For this review, use the dimensioned drawing (mm, ordinates from the lowest corner) and the shaded views. A direction names the side the tool comes from. Coordinates: 2 decimals unless noted, no trailing zeros. Loops run counter-clockwise (first coordinate to the right, second up) from the corner with the lowest first, then second, coordinate; pieces in that order, holes last. Notation, with made-up numbers: M 81,-29.5 L 126,-29.5 A8 ccw 126,-15.5 Z; hole C 9.25,64 d7. An arc over 180 degrees is marked long. Write item = value, one per line.
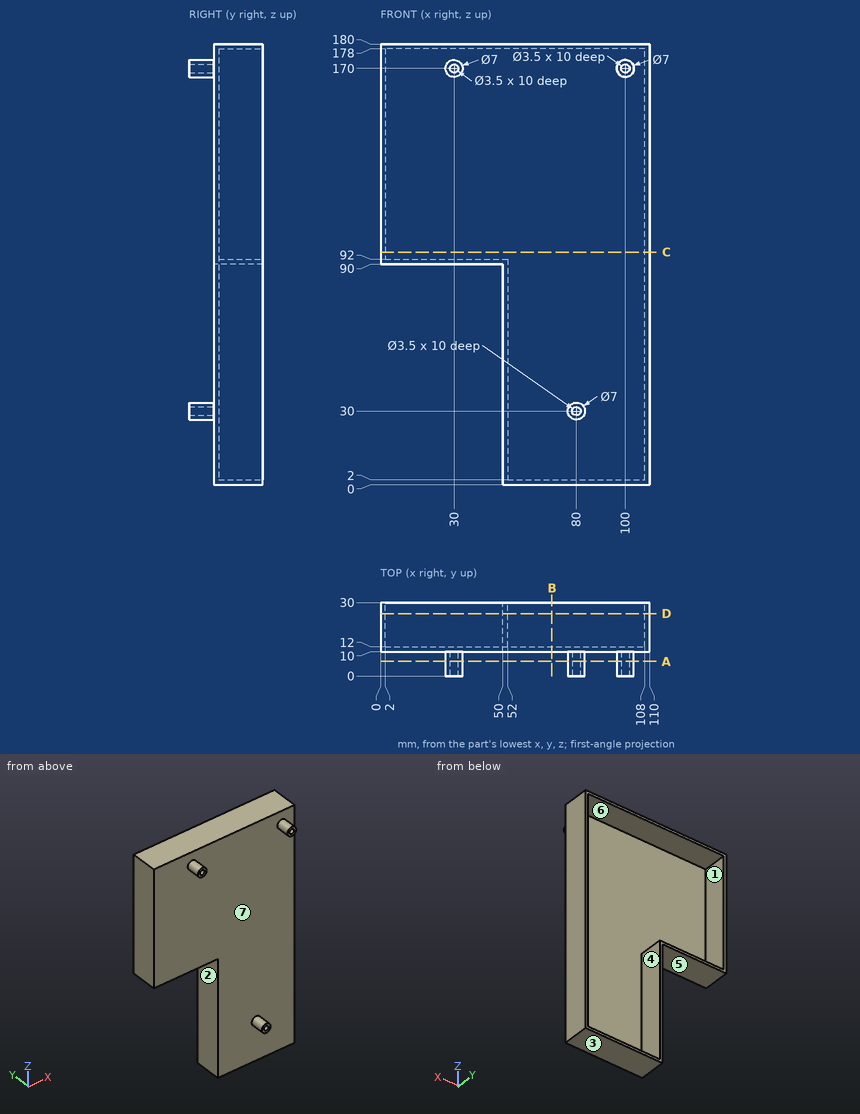
Q1. Machinability: for the marked faces 1, 2 and 3, which of the approach directions +Z, -Z, +X, -X, +Y, -Y give a long, thin tool a straight path to every point of the face, cutting with its end or side? Answer none if there is none.
Solved:
face_1 = +Y
face_2 = -Z, -X, +Y, -Y
face_3 = -Z, +X, -X, +Y, -Y
Q2. Add section D-D (y = 25.5). Write out the cut boundary in (x, z).
Solved:
outline = M 0,90 L 50,90 L 50,0 L 110,0 L 110,180 L 0,180 Z; hole M 2,92 L 52,92 L 52,2 L 108,2 L 108,178 L 2,178 Z
Q3. For pin 1 Ø1 at (x, z) = (80, 29.5) entering from -Y; pin 2 Ø4 at (x, z) = (30, 170) entering from +Y; pin 3 Ø6 at (x, y) = (36, 17.5) entering from -Z, all flat-tipped, find the tip position at first contact; note any pin that passes through.
Solved:
pin_1 = 10
pin_2 = 12
pin_3 = 90
Q4. For line 1 along X through (y, z) = (3.25, 170); line 2 along Z through (x, y) = (100, 5.75); line 3 along Z through (x, y) = (80, 7), list the stretches that pass through material, from the lowest coordinate up.
Solved:
line_1 = 26.5 to 28.25, 31.75 to 33.5, 96.5 to 98.25, 101.75 to 103.5
line_2 = 166.5 to 168.25, 171.75 to 173.5
line_3 = 26.5 to 28.25, 31.75 to 33.5
Q5. Add section C-C (z = 95). Write out the cut boundary in (x, y).
Solved:
outline = M 0,10 L 110,10 L 110,30 L 108,30 L 108,12 L 2,12 L 2,30 L 0,30 Z
Q6. Add section B-B (x = 70). Write out the cut boundary in (y, z), and give its area (3 significant figures).
Solved:
outline = M 10,0 L 30,0 L 30,2 L 12,2 L 12,178 L 30,178 L 30,180 L 10,180 Z
area = 432 mm²
Q7. Draft analysis for pull direction Z (two halves, no side actions). For the marked faces 4, 5, 6 and 7, state which applies: +Z half, -Z half, draft (parallel to the pull), parting line (faces both ways), or undercut.
Solved:
face_4 = undercut
face_5 = -Z half
face_6 = undercut
face_7 = draft
Q8. Add section A-A (y = 6). Write out the cut boundary in (x, z).
Solved:
outline = C 30,170 d7; C 80,30 d7; C 100,170 d7; hole C 30,170 d3.5; hole C 80,30 d3.5; hole C 100,170 d3.5
